Verification items for the finished model (mm, model axes). A direction names the side the tool comes from. Round coordinates to 2 decimals unless told otherwise and drop trailing zeros. Write each loop counter-clockwise with the first axis right and the second up, starting at its lowest first coordinate (ties: lowest second). Pieces come first, ordered by that corner, then holes. Notation, with made-up numbers: M 61,-1.5 L 103,-1.5 A13 cw 103,19.5 Z; hole C 64,-9.5 d10. An arc over 180 degrees is marked long. Answer in a Markdown table with one row per item. Add a question column.
1. Sectioned sample at A-A on y = 8.25. Record the cut outline in (x, z) (3 decimals), plus the area to 3 significant figures.
2. Go/stop test with flat-tipped pins: pin 1 Ø4 at (y, z) = (4, -10) entering from -X (3 decimals); pin 2 Ø4 at (x, y) = (-39, 13) entering from +Z. Record where each tip stops, or that it passes through.
3. Draft check along Y on faces 3 (the cylindrical face through (-8.05, 12.2, -10.99)), 4 (the flat face through (-23, 0, -46)), 5 (the cylindrical face through (-24.146, 10.717, -34.314)), 6 (the flat face through (0, 14, -39)). Enter one of: pulls with the +Y half, pulls with the -Y half, needs draft (parallel to the pull), parting line crosses it, or undercut.
4. Set-up check for faces 1 (the flat face through (-35, 10, -25.4)), 2 (the flat face through (-8, 9, 0)): record each of +Z, -Z, +X, -X, +Y, -Y from which the full face is reachable in a straight line by a thin tool's end or side.
5. Sectioned sample at C-C on z = -63. Record the cut outline in (x, y) (3 decimals).
6. Material ranges on probe 1 along X at (y, z) = (6.5, -50.8) (3 decimals); probe 2 along Z at (x, y) = (-38.1, 9.5) (3 decimals); probe 3 along Z at (x, y) = (-38.1, 14) (3 decimals), recorded low to high.
7. Sectioned sample at D-D on z = -52. Count the separate pieces of the cut face and the enclosed holes in it, plus the area to 3 significant figures.
8. Sectioned sample at B-B on x = -12.7. Record the cut outline in (y, z) (3 decimals).
Autodesk Inventor part; units mm, degrees
ref_plane "YZ Plane" through (0, 0, 0) normal (1, 0, 0) x (0, 1, 0)
ref_plane "XZ Plane" through (0, 0, 0) normal (0, 1, 0) x (-1, 0, 0)
ref_plane "XY Plane" through (0, 0, 0) normal (0, 0, 1) x (1, 0, 0)
sketch "Sketch1" plane through (0, 0, 0) normal (0, 1, 0) x (-1, 0, 0)
  line L0 (0, 0) -> (47.625, 0)
  line L1 (47.625, 0) -> (47.625, -76.2)
  line L2 (47.625, -76.2) -> (0, -76.2)
  line L3 (0, -76.2) -> (0, 0)
  dimension "d0" = 47.625
  dimension "d1" = 76.2
extrude "Extrusion1" add sketch "Sketch1" along normal blind 19.05
sketch "Sketch2" plane through (-47.625, 0, -76.2) normal (-1, 0, 0) x (0, 0, 1)
  line L0 (0, 0) -> (0, 19.05)
  line L1 (0, 19.05) -> (76.2, 19.05)
  line L2 (76.2, 0) -> (0, 0)
  line L3 (48.9575, 0) -> (51.7141, 0)
  line L4 (51.7141, 0) -> (51.7141, 9.525)
  line L5 (51.7141, 9.525) -> (48.9575, 9.525)
  line L6 (48.9575, 9.525) -> (48.9575, 0)
  line L7 (0, 0) -> (76.2, 0)
  line L8 (0, 9.525) -> (50.8, 9.525)
  line L9 (0, 9.525) -> (25.4, 9.525)
  line L10 (76.2, 0) -> (76.2, 19.05)
  line L11 (50.8, 9.525) -> (38.1, 9.525)
  line L12 (25.4, 9.525) -> (12.7, 9.525)
  circle A0 centre (38.1, 9.525) radius 3.9688
  circle A1 centre (12.7, 9.525) radius 3.9688
  point P0 (53.975, 9.525)
  point P1 (53.975, 0)
  dimension "d8" = 50.8
  dimension "d9" = 25.4
  dimension "d10" = 7.9375
  dimension "d11" = 7.9375
sketch "Sketch3" plane through (-47.625, 0, -76.2) normal (-1, 0, 0) x (0, 0, 1)
  line L0 (76.2, 19.05) -> (50.8, 19.05)
  line L1 (50.8, 19.05) -> (50.8, 0)
  line L2 (50.8, 0) -> (76.2, 0)
  line L3 (76.2, 0) -> (76.2, 19.05)
  point P0 (76.2, 0)
  dimension "d21" = 25.4
  dimension "d27" = 19.05
extrude "Extrusion3" cut sketch "Sketch3" against normal blind 31.75
fillet "Fillet4" radius 6.35 1 edges at (-15.875, 9.525, -25.4)
extrude "Extrusion4" cut sketch "Sketch2" against normal through all contours A1 L8 | L8 A1 | A0 L8 | L8 A0
sketch "Sketch5" plane through (-15.875, 0, -76.2) normal (-1, 0, 0) x (0, 0, 1)
  line L0 (50.8, 0) -> (50.8, 19.05)
  line L1 (76.2, 19.05) -> (76.2, 0)
  line L2 (76.2, 9.525) -> (63.5, 9.525)
  circle A0 centre (63.5, 9.525) radius 3.175
  dimension "d28" = 12.7
  dimension "d29" = 6.35
extrude "Extrusion5" cut sketch "Sketch5" along normal mid plane 44.45
sketch "Sketch7" plane through (0, 19.05, 0) normal (0, 1, 0) x (1, 0, 0)
  line L0 (-47.625, 25.4) -> (-47.625, 50.8)
  line L1 (-47.625, 50.8) -> (-38.1, 50.8)
  circle A0 centre (-38.1, 50.8) radius 3.175
  line L2 (-38.1, 50.8) -> (-12.7, 50.8)
  circle A1 centre (-12.7, 50.8) radius 3.175
  point P0 (0, 0)
  dimension "d37" = 25.4
  dimension "d38" = 9.525
  dimension "d39" = 6.35
  dimension "d40" = 25.4
  dimension "d41" = 6.35
extrude "Extrusion7" cut sketch "Sketch7" against normal blind 25.4
properties part number "34Assembly"
Geometry check:
| question | item | result |
|---|---|---|
| 1 | outline | M -47.625,-76.2 L 0,-76.2 L 0,-67.258 L -47.625,-67.258 Z; M -47.625,-59.742 L 0,-59.742 L 0,-41.858 L -47.625,-41.858 Z; M -47.625,-34.342 L 0,-34.342 L 0,-15.608 L -15.875,-15.608 L -15.875,-19.05 A6.35 cw -22.225,-25.4 L -47.625,-25.4 Z; M -15.875,-9.792 L 0,-9.792 L 0,0 L -15.875,0 Z; hole C -38.1,-50.8 d6.35; hole C -12.7,-50.8 d6.35 |
| 1 | area | 1,960 mm2 |
| 2 | pin 1 | stops at x = -15.875 |
| 2 | pin 2 | stops at z = -25.4 |
| 3 | face 3 | undercut |
| 3 | face 4 | pulls with the -Y half |
| 3 | face 5 | undercut |
| 3 | face 6 | needs draft |
| 4 | face 1 | +Z, -X, +Y, -Y |
| 4 | face 2 | +Z, +X, -X, +Y, -Y |
| 5 | outline | M -47.625,0 L 0,0 L 0,5.588 L -47.625,5.588 Z; M -47.625,13.462 L 0,13.462 L 0,19.05 L -47.625,19.05 Z |
| 6 | probe 1 | x = -47.625 to -41.275, -34.925 to -15.875, -9.525 to 0 |
| 6 | probe 2 | z = -76.2 to -67.469, -59.531 to -53.975, -47.625 to -42.069, -34.131 to -25.4 |
| 6 | probe 3 | z = -76.2 to -53.975, -47.625 to -25.4 |
| 7 | separate pieces | 3 |
| 7 | enclosed holes | 0 |
| 7 | area | 683 mm2 |
| 8 | outline | M 0,-76.2 L 19.05,-76.2 L 19.05,-53.975 L 0,-53.975 Z; M 0,-47.625 L 19.05,-47.625 L 19.05,0 L 0,0 Z; hole C 9.525,-63.5 d7.938; hole C 9.525,-38.1 d7.938; hole C 9.525,-12.7 d6.35 |
